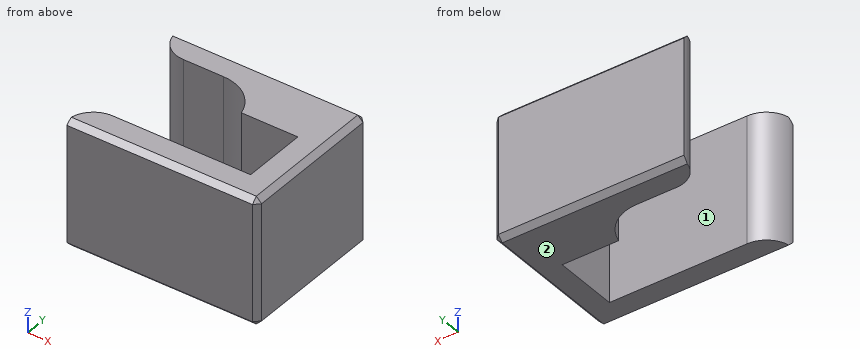
```python
from build123d import *

# Parameters (mm, degrees)
F1_DEPTH = 6
F2_SIZE  = 0.5


with BuildPart() as f1:
    # F0 (on Top) → F1 (new body, symmetric)
    with BuildSketch(Plane.XY):
        with BuildLine():
            Line((9, 7.05), (-9, 7.05))
            ThreePointArc((-9, 7.05), (-8.267767, 5.282233), (-6.5, 4.55))
            Line((-6.5, 4.55), (-2.70464, 4.55))
            ThreePointArc((-2.70464, 4.55), (-0.25515, 3.712278), (1.168343, 1.55))
            Line((1.168343, 1.55), (6.5, 1.55))
            Line((6.5, 1.55), (6.5, -4.55))
            Line((6.5, -4.55), (-6.5, -4.55))
            ThreePointArc((-6.5, -4.55), (-8.267767, -5.282233), (-9, -7.05))
            Line((-9, -7.05), (9, -7.05))
            Line((9, -7.05), (9, 7.05))
        make_face()
    extrude(amount=F1_DEPTH, both=True)

    # F2
    f2_edges = [f1.edges().sort_by_distance(p)[0] for p in [
        (9, 7.05, 0),
        (9, -7.05, 0),
        (9, 0, 6),
        (9, 0, -6),
        (0, 7.05, -6),
        (0, 7.05, 6),
        (0, -7.05, 6),
        (0, -7.05, -6),
    ]]
    chamfer(f2_edges, length=F2_SIZE)


with BuildPart() as f3_1:
    # F3: copy of F1
    add(f1.part.moved(Location((26.4, 0, 0))))


solid = f1.part
```
For this review, take the finished solid that the model builds, in its own axes (mm). Face numbers are marked on the shaded views. A direction names the side the tool comes from. Give positions to 0.01 mm unless a question says otherwise; leave off trailing zeros. Loops run counter-clockwise (first coordinate to the right, second up) from the corner with the lowest first, then second, coordinate; pieces in that order, holes last. Notation, with made-up numbers: M 14.25,62.25 L 49.25,62.25 A18 cw 49.25,92.25 Z; hole C 49.25,56 d4. An arc over 180 degrees is marked long. One line per item, written item: value. Start each with the question number.
Q1. Machinability: for the marked faces 1 and 2, which of the approach directions +Z, -Z, +X, -X, +Y, -Y give a long, thin tool a straight path to every point of the face, cutting with its end or side? Answer none if there is none.
Q2. Add section C-C (z = -3). Give the boundary of the cut face in (x, y), and give its area (3 significant figures).
Q3. Add section D-D (x = -3.25). Give the boundary of the cut face in (y, z), and give its area (3 significant figures).
Q4. Add section B-B (y = -1). Give the boundary of the cut face in (x, z), and give its area (4 significant figures).
Q5. Add section A-A (x = 4). Give the boundary of the cut face in (y, z).
Q6. For L1, parallel to Y at x = -4, z = 4.25; L2, parallel to X at y = -2.5, z = -5, list the stretches that pass through material, from the lowest coordinate up.
Q7. Clearance check with flat-ended pins moving along their axes: pin 1 Ø1.8 at (y, z) = (-2, 2) entering from -X; pin 2 Ø4 at (x, y) = (2, -1.5) entering from -Z. State where each tip first meets the part, or that it passes through.
Reply:
1. face 1: +Z, -Z, -X
1. face 2: -Z, +X, -X, +Y, -Y
2. outline: M -9,-7.05 L 8.5,-7.05 L 9,-6.55 L 9,6.55 L 8.5,7.05 L -9,7.05 A2.5 ccw -6.5,4.55 L -2.7,4.55 A4 cw 1.17,1.55 L 6.5,1.55 L 6.5,-4.55 L -6.5,-4.55 A2.5 ccw Z
2. area: 129 mm²
3. outline: M -7.05,-5.5 L -6.55,-6 L -4.55,-6 L -4.55,6 L -6.55,6 L -7.05,5.5 Z; M 4.55,-6 L 6.55,-6 L 7.05,-5.5 L 7.05,5.5 L 6.55,6 L 4.55,6 Z
3. area: 59.5 mm²
4. outline: M 6.5,-6 L 8.5,-6 L 9,-5.5 L 9,5.5 L 8.5,6 L 6.5,6 Z
4. area: 29.75 mm²
5. outline: M -7.05,-5.5 L -6.55,-6 L -4.55,-6 L -4.55,6 L -6.55,6 L -7.05,5.5 Z; M 1.55,-6 L 6.55,-6 L 7.05,-5.5 L 7.05,5.5 L 6.55,6 L 1.55,6 Z
6. L1: -7.05 to -4.55, 4.55 to 7.05
6. L2: 6.5 to 9
7. pin 1: x = 6.5
7. pin 2: through
